Input: dimensioned drawing with shaded views. Units: mm. Origin: part minimum x, y, z. A direction names the side the tool comes from. Round coordinates to 2 decimals unless told otherwise and drop trailing zeros. Loops run counter-clockwise (first coordinate to the right, second up) from the corner with the lowest first, then second, coordinate; pieces in that order, holes last. Notation, with made-up numbers: M 56.25,69 L 85.25,69 A12 cw 85.25,73 Z; hole C -18.75,45 d9. An arc over 180 degrees is marked long. Put each result on its own line as item: value. Start each with the question number.
1) Section C-C on z = 1.5. Output: boundary loops of the cut face in (x, y) (3 decimals).
2) Reachability of the marked faces 1 and 2 from +Z, -Z, +X, -X, +Y, -Y: full face, straight path, thin tool, end or side. Return the list, or none.
3) Section D-D on y = 13.5. Output: boundary loops of the cut face in (x, z), plus the area to 3 significant figures.
4) Line query: probe 1 along Y at (x, z) = (127, 2.9) (3 decimals); probe 2 along X at (y, z) = (6, 3.25); probe 3 along Y at (x, z) = (11, 2.5). Output: solid intervals per line, ascending.
5) Section B-B on y = 2.5. Output: boundary loops of the cut face in (x, z), plus the area to 3 significant figures.
6) Section A-A on x = 143. Output: boundary loops of the cut face in (y, z) (3 decimals).
7) Pin query (flat end, axial travel): pin 1 (6 mm diameter, centred on x = 124, y = 12, fed in from +Z); pin 2 (4 mm diameter, centred on y = 6, z = 8.5, fed in from +X); pin 3 (4.5 mm diameter, centred on x = 127, y = 7.5, fed in from +Z). Return the tip coordinate at first contact, or that it passes through.
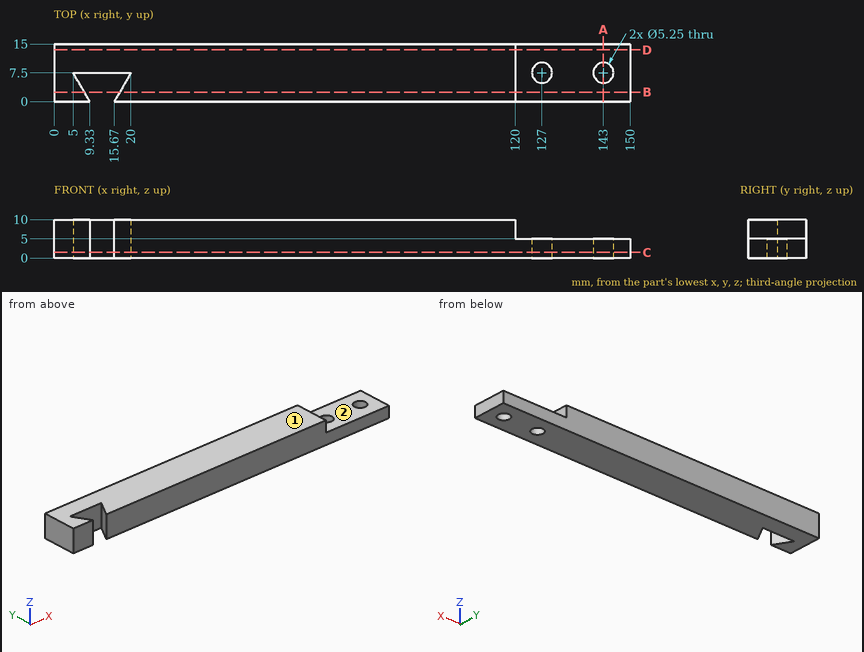
Geometry results:
1. outline: M 0,0 L 9.33,0 L 5,7.5 L 20,7.5 L 15.67,0 L 150,0 L 150,15 L 0,15 Z; hole C 127,7.5 d5.25; hole C 143,7.5 d5.25
2. face 1: +Z, +X, -X, +Y, -Y
2. face 2: +Z, +X, +Y, -Y
3. outline: M 0,0 L 150,0 L 150,5 L 120,5 L 120,10 L 0,10 Z
3. area: 1,350 mm²
4. probe 1: y = 0 to 4.875, 10.125 to 15
4. probe 2: x = 0 to 5.87, 19.13 to 124.85, 129.15 to 140.85, 145.15 to 150
4. probe 3: y = 7.5 to 15
5. outline: M 0,0 L 7.89,0 L 7.89,10 L 0,10 Z; M 17.11,0 L 150,0 L 150,5 L 120,5 L 120,10 L 17.11,10 Z
5. area: 1,260 mm²
6. outline: M 0,0 L 4.875,0 L 4.875,5 L 0,5 Z; M 10.125,0 L 15,0 L 15,5 L 10.125,5 Z
7. pin 1: stops at z = 5
7. pin 2: stops at x = 120
7. pin 3: passes through
